```python
from build123d import *

# Parameters (mm, degrees)
F0_W     = 4.8
F0_H     = 2.52
F1_DEPTH = 12.5
F2_W     = 1.5
F2_H     = 7
F3_DEPTH = 1
F4_R     = 6.25
F5_DEPTH = 4
F7_DEPTH = 2.52
F9_DEPTH = 2.52


with BuildPart() as f1:
    # F0 (on Top) → F1 (new body)
    with BuildSketch(Plane.XY):
        Polygon((25.5896202285, 7.390901965), (3.0896202285, 7.390901965), (3.0896202285, 3.290901965), (3.0896202285, 0.770901965), (3.0896202285, -17.609098035), (25.5896202285, -17.609098035), (25.5896202285, 0.770901965), (25.5896202285, 3.290901965), align=None)
        with Locations((27.9896202285, 2.030901965)):
            Rectangle(F0_W, F0_H)
        with Locations((0.6896202285, 2.030901965)):
            Rectangle(F0_W, F0_H)
    extrude(amount=F1_DEPTH)

    # F2 (on face) → F3 (cut)
    with BuildSketch(Plane.YZ.offset(25.5896202285)):
        with Locations((-9.979098035, 6.5)):
            Rectangle(F2_W, F2_H)
    extrude(amount=-F3_DEPTH, mode=Mode.SUBTRACT)

    # F4 (on face) → F5 (join)
    with BuildSketch(Plane(origin=(0, 7.390901965, 0), x_dir=(-1, 0, 0), z_dir=(0, 1, 0))):
        with Locations((-19.3396202285, 6.25)):
            Circle(F4_R)
    extrude(amount=F5_DEPTH)

    # F6 (on face) → F7 (cut, through all)
    with BuildSketch(Plane(origin=(0, 3.290901965, 0), x_dir=(-1, 0, 0), z_dir=(0, 1, 0))):
        with BuildLine():
            Line((-30.3896202285, 5.7453945725), (-28.8729703096, 5.7453945725))
            ThreePointArc((-28.8729703096, 5.7453945725), (-29.0096060883, 6.2446820853), (-28.8782882995, 6.7453945725))
            Line((-28.8782882995, 6.7453945725), (-30.3896202285, 6.7453945725))
            Line((-30.3896202285, 6.7453945725), (-30.3896202285, 5.7453945725))
        make_face()
        with BuildLine():
            Line((-28.8729703096, 6.7453945725), (-28.8729703096, 5.7453945725))
            ThreePointArc((-28.8729703096, 5.7453945725), (-27.7482297936, 5.2847668465), (-27.0096202285, 6.25))
            ThreePointArc((-27.0096202285, 6.25), (-27.7533665173, 7.2166095569), (-28.8782882995, 6.7453945725))
            Line((-28.8782882995, 6.7453945725), (-28.8729703096, 6.7453945725))
        make_face()
        with BuildLine():
            ThreePointArc((-28.8782882995, 6.7453945725), (-29.0096060883, 6.2446820853), (-28.8729703096, 5.7453945725))
            Line((-28.8729703096, 5.7453945725), (-28.8729703096, 6.7453945725))
            Line((-28.8729703096, 6.7453945725), (-28.8782882995, 6.7453945725))
        make_face()
    extrude(amount=-F7_DEPTH, mode=Mode.SUBTRACT)

    # F8 (on face) → F9 (cut, through all)
    with BuildSketch(Plane(origin=(0, 3.290901965, 0), x_dir=(-1, 0, 0), z_dir=(0, 1, 0))):
        with BuildLine():
            ThreePointArc((0.1964051753, 5.75), (0.2963055978, 5.9911809549), (0.3303797715, 6.25))
            ThreePointArc((0.3303797715, 6.25), (0.2963055978, 6.5088190451), (0.1964051753, 6.75))
            Line((0.1964051753, 6.75), (-0.2896202285, 6.75))
            Line((-0.2896202285, 6.75), (-0.2896202285, 5.75))
            Line((-0.2896202285, 5.75), (0.1964051753, 5.75))
        make_face()
        with BuildLine():
            ThreePointArc((0.1964051753, 6.75), (0.2963055978, 6.5088190451), (0.3303797715, 6.25))
            ThreePointArc((0.3303797715, 6.25), (0.2963055978, 5.9911809549), (0.1964051753, 5.75))
            Line((0.1964051753, 5.75), (1.7103797715, 5.75))
            Line((1.7103797715, 5.75), (1.7103797715, 6.75))
            Line((1.7103797715, 6.75), (0.1964051753, 6.75))
        make_face()
        with BuildLine():
            Line((-0.2896202285, 6.75), (0.1964051753, 6.75))
            ThreePointArc((0.1964051753, 6.75), (-1.6696202285, 6.25), (0.1964051753, 5.75))
            Line((0.1964051753, 5.75), (-0.2896202285, 5.75))
            Line((-0.2896202285, 5.75), (-0.2896202285, 6.75))
        make_face()
    extrude(amount=-F9_DEPTH, mode=Mode.SUBTRACT)


solid = f1.part
```
Can you work these out from the model? Positions are in its coordinate system, mm. A direction names the side the tool comes from. Coordinates: 2 decimals unless noted, no trailing zeros. Loops run counter-clockwise (first coordinate to the right, second up) from the corner with the lowest first, then second, coordinate; pieces in that order, holes last. Notation, with made-up numbers: M 76.5,-32.5 L 84.5,-32.5 A23 ccw 84.5,-4.5 Z; hole C 55,57 d3. An arc over 180 degrees is marked long. Put each result on its own line as item: value. Start each with the question number.
(1) Will these pins go through, and if not, where does the flat tip stop? pin 1 Ø6 at (x, z) = (3, 5.5) entering from +Y; pin 2 Ø2.5 at (x, z) = (0.67, 6.25) entering from -Y; pin 3 Ø2 at (y, z) = (5, 9) entering from +X.
(2) Imagine slicing it at C-C on x = 5. List the corners of the cut face in (y, z) for me, and give its area (4 significant figures).
(3) We'd pull the mould along Z, two halves only. Please class faces 5 (the face through (14, -5, 12.5)), 6 (the face through (-1.71, 2, 10)), 7 (the face through (25, -10, 10)), 8 (the face through (-1, 2, 5.75)): +Z half, -Z half, draft (parallel to the pull), parting line (faces both ways), or undercut.
(4) Imagine slicing it at A-A on y = 2.75. List the corners of the cut face in (x, z) for me, and give its area (3 significant figures).
(5) Imagine slicing it at D-D on x = 14. List the corners of the cut face in (y, z) for me, and give its area (3 significant figures).
(6) I need wall thicknesses on probe 1 along Y at (x, z) = (15.5, 0.75); probe 2 along X at (y, z) = (6.5, 1.75); probe 3 along Y at (x, z) = (28, 2.25). Which ranges of each line are inside material? Lowest first, please.
(7) Imagine slicing it at B-B on z = 2. List the corners of the cut face in (x, y) for me, and give its area (3 significant figures).
(8) Which directions (+Z, -Z, +X, -X, +Y, -Y) give clear straight access to the entire face, cutting with the end or side of a thin tool? Please do faces 1 (the face through (25, -10.729, 6)), 2 (the face through (30, 2, 5.745)), 3 (the face through (2, 0.771, 6)), 4 (the face through (24, 7.391, 11)).
Worked answers:
1. pin 1: stops at y = 7.39
1. pin 2: stops at y = 0.77
1. pin 3: stops at x = 25.59
2. outline: M -17.61,0 L 7.39,0 L 7.39,12.5 L -17.61,12.5 Z
2. area: 312.5 mm2
3. face 5: +Z half
3. face 6: draft
3. face 7: undercut
3. face 8: undercut
4. outline: M -1.71,0 L 30.39,0 L 30.39,5.75 L 28.87,5.75 A1 cw long 28.88,6.75 L 30.39,6.75 L 30.39,12.5 L -1.71,12.5 L -1.71,6.75 L -0.2,6.75 A1 cw long -0.2,5.75 L -1.71,5.75 Z
4. area: 392 mm2
5. outline: M -17.61,0 L 7.39,0 L 7.39,3 L 11.39,3 L 11.39,9.5 L 7.39,9.5 L 7.39,12.5 L -17.61,12.5 Z
5. area: 338 mm2
6. probe 1: y = -17.61 to 7.39
6. probe 2: x = 3.09 to 25.59
6. probe 3: y = 0.77 to 3.29
7. outline: M -1.71,0.77 L 3.09,0.77 L 3.09,-17.61 L 25.59,-17.61 L 25.59,0.77 L 30.39,0.77 L 30.39,3.29 L 25.59,3.29 L 25.59,7.39 L 23.92,7.39 L 23.92,11.39 L 14.76,11.39 L 14.76,7.39 L 3.09,7.39 L 3.09,3.29 L -1.71,3.29 Z
7. area: 623 mm2
8. face 1: +X
8. face 2: +X, +Y, -Y
8. face 3: +Z, -Z, -X, -Y
8. face 4: +Z, +X, +Y
